Could you check a few things on this model? Use its own coordinates, in mm. A direction names the side the tool comes from. Give positions to 0.01 mm unless a question says otherwise; leave off trailing zeros. Loops run counter-clockwise (first coordinate to the right, second up) from the corner with the lowest first, then second, coordinate; pieces in that order, holes last. Notation, with made-up numbers: (28, -6) -> (41, -6) arc R17 cw to (41, 22) -> close; hole circle Ø3 at (15, 42). An arc over 180 degrees is marked (long way). Write each question's results on one line, items separated by ' | '. Start each with the question number.
Q1. Which directions (+Z, -Z, +X, -X, +Y, -Y) give clear straight access to the entire face, cutting with the end or side of a thin tool? Please do faces 1 (the face through (0, 177, 19.05)), 2 (the face through (17.462, 177, 0)).
Q2. If we section it at A-A, the plane x = 0: Give the number of separate pieces and of enclosed holes in the cut face, plus the area to 3 significant figures.
Q3. We'd pull the mould along Z, two halves only. Please class faces 3 (the face through (0, 177, 17.462)), 4 (the face through (0, 177, -19.05)), 5 (the face through (-2, 358.775, 18)): released by +Z, released by -Z, zero draft, split by the parting line, or undercut.
Q4. If I drill on line 1 along Z through (x, y) = (0, 106); line 2 along Y through (x, z) = (-4, 17.5) (3 decimals), over which ranges is the centre line in solid material (lowest first)?
Q5. If we section it at C-C, the plane y = 274: List the corners of the cut face in (x, z) for me, plus the area to 3 significant figures.
from build123d import *

# Parameters (mm, degrees)
SKETCH1_W           = 38.1
SKETCH1_H           = 38.1
SKETCH1_W_2         = 34.925
SKETCH1_H_2         = 34.925
BOSS_EXTRUDE1_DEPTH = 358.775
SKETCH2_R           = 14.2875
SKETCH2_R_2         = 2.5527
SKETCH2_R_3         = 14.294919975
CUT_EXTRUDE1_DEPTH  = 362.294911568


with BuildPart() as part:
    # Sketch1 → Boss-Extrude1 (new body)
    with BuildSketch(Plane(origin=(0, 0, 0), x_dir=(1, 0, 0), z_dir=(0, 1, 0))):
        Rectangle(SKETCH1_W, SKETCH1_H)
        Rectangle(SKETCH1_W_2, SKETCH1_H_2, mode=Mode.SUBTRACT)
    extrude(amount=BOSS_EXTRUDE1_DEPTH)

    # Sketch2 → Cut-Extrude1 (cut, through all)
    with BuildSketch(Plane(origin=(0, 0, -19.05), x_dir=(-1, 0, 0), z_dir=(0, 0, -1))):
        with Locations((0, 333.375)):
            Circle(SKETCH2_R)
        with Locations((-11.90625, 5.311170072)):
            Circle(SKETCH2_R_2)
        with Locations((-11.90625, 46.555629928)):
            Circle(SKETCH2_R_2)
        with Locations((11.90625, 46.555629928)):
            Circle(SKETCH2_R_2)
        with Locations((11.90625, 5.311170072)):
            Circle(SKETCH2_R_2)
        with Locations((0, 25.9334)):
            Circle(SKETCH2_R_3)
    extrude(amount=-CUT_EXTRUDE1_DEPTH, mode=Mode.SUBTRACT)


solid = part.part
Final values:
1) face 1: +Z, +X, -X, +Y, -Y | face 2: +Y, -Y
2) separate pieces: 6 | enclosed holes: 0 | area: 958 mm²
3) face 3: undercut | face 4: released by -Z | face 5: zero draft
4) line 1: z = -19.05 to -17.46, 17.46 to 19.05 | line 2: y = 0 to 12.21, 39.657 to 319.659, 347.091 to 358.775
5) outline: (-19.05, -19.05) -> (19.05, -19.05) -> (19.05, 19.05) -> (-19.05, 19.05) -> close; hole (-17.46, -17.46) -> (17.46, -17.46) -> (17.46, 17.46) -> (-17.46, 17.46) -> close | area: 232 mm²
